Autodesk Inventor part; units mm, degrees
ref_plane "YZ Plane" through (0, 0, 0) normal (1, 0, 0) x (0, 1, 0)
ref_plane "XZ Plane" through (0, 0, 0) normal (0, 1, 0) x (-1, 0, 0)
ref_plane "XY Plane" through (0, 0, 0) normal (0, 0, 1) x (1, 0, 0)
sketch "Sketch1" plane through (0, 0, 0) normal (0, 0, 1) x (1, 0, 0)
  line L0 (0, 0) -> (31.75, 0)
  line L1 (31.75, 0) -> (31.75, 6.35)
  line L2 (31.75, 25.4) -> (28.575, 25.4) construction
  line L3 (0, 25.4) -> (0, 6.35) construction
  line L4 (0, 6.35) -> (3.175, 6.35)
  line L5 (3.175, 6.35) -> (3.175, 25.4)
  line L6 (28.575, 25.4) -> (28.575, 6.35)
  line L7 (28.575, 6.35) -> (31.75, 6.35)
  line L8 (0, 6.35) -> (0, 0)
  line L9 (3.175, 25.4) -> (0, 25.4) construction
  line L10 (28.575, 25.4) -> (3.175, 25.4)
  line L11 (31.75, 6.35) -> (31.75, 25.4) construction
  dimension "d0" = 31.75
  dimension "d1" = 25.4
  dimension "d2" = 6.35
  dimension "d3" = 3.175
extrude "Extrusion1" add sketch "Sketch1" along normal blind 98.425
sketch "Sketch2" plane through (3.175, 25.4, 0) normal (0, 1, 0) x (1, 0, 0)
  line L0 (0, -98.425) -> (25.4, -98.425)
  line L1 (25.4, 0) -> (25.4, -98.425)
  line L2 (25.4, 0) -> (0, 0)
  line L3 (0, 0) -> (0, -98.425)
  point P0 (-3.175, 0)
  point P1 (12.7, -85.725)
  point P2 (12.7, -12.7)
  dimension "d6" = 12.7
  dimension "d7" = 12.7
  dimension "d8" = 12.7
  dimension "d9" = 12.7
hole "Hole1" at (15.875, 25.4, 85.725) at (15.875, 25.4, 12.7) direction (0, -1, 0) diameter 6.35 end through all counterbore diameter 9.525 counterbore depth 6.35
properties part number "8 ball plastic slider"
Input: part model. Units: mm. Frame: model coordinates. A direction names the side the tool comes from. Coordinates: 2 decimals unless noted, no trailing zeros. Write each loop counter-clockwise with the first axis right and the second up, starting at its lowest first coordinate (ties: lowest second). Pieces come first, ordered by that corner, then holes. Notation, with made-up numbers: M -9,-2.75 L -3,-2.75 A14 ccw -3,5.25 Z; hole C -32.5,-12 d2. An arc over 180 degrees is marked long. Answer as a JSON object with one key per item and string values. Group by question number.
(1) Set-up query: faces 5 (the face through (18.77, 22.18, 8.92)), 6 (the face through (3.175, 16, 49)), 7 (the face through (16, 0, 49)), 8 (the face through (30, 6.35, 49)). Return all of +Z, -Z, +X, -X, +Y, -Y with unobstructed straight access to the full face (end or side cutting, diameter ignored); none if empty.
(2) Ray query, line 1 along Z through (x, y) = (15.5, 23) (3 decimals); line 2 along Z through (x, y) = (11.5, 24) (3 decimals); line 3 along X through (y, z) = (13.25, 12.7) (3 decimals). Return the intervals inside material, ascending. Write a range as [from, to].
(3) Section D-D on x = 30.5. Output: boundary loops of the cut face in (y, z) (3 decimals), plus the area to 3 significant figures.
(4) Section B-B on y = 5. Output: boundary loops of the cut face in (x, z) (3 decimals), plus the area to 3 significant figures.
(5) Section C-C on z = 25. Output: boundary loops of the cut face in (x, y) (3 decimals), plus the area to 3 significant figures.
(6) Contact query for flat-ended pins moving along their axis: P1, Ø1.5, axis at x = 8, y = 3, coming from the -Z side; P2, Ø5, axis at y = 22, z = 84, coming from the +X side (3 decimals); P3, Ø1.6, axis at x = 30, z = 70.5, coming from the +Y side; P4, Ø8.5, axis at x = 15.875, z = 12.7, coming from the +Y side. Output: stop coordinate, or through.
(7) Mould query, pull axis Z, two halves, no side actions, for faces 1 (the face through (31.75, 3, 49)), 2 (the face through (16, 13, 98.425)), 3 (the face through (18.773, 22.181, 81.946)), 4 (the face through (15.735, 9.392, 9.528)). Classes: pulls with the +Z half, pulls with the -Z half, needs draft (parallel to the pull), parting line crosses it, or undercut.
Result set:
{
 "1": {"face 5": "+Y", "face 6": "+Z, -Z, -X, +Y", "face 7": "+Z, -Z, +X, -X, -Y", "face 8": "+Z, -Z, +X, +Y"},
 "2": {"line 1": "z = [0, 7.952], [17.448, 80.977], [90.473, 98.425]", "line 2": "z = [0, 10.818], [14.582, 83.843], [87.607, 98.425]", "line 3": "x = [3.175, 12.7], [19.05, 28.575]"},
 "3": {"outline": "M 0,0 L 6.35,0 L 6.35,98.425 L 0,98.425 Z", "area": "625 mm2"},
 "4": {"outline": "M 0,0 L 31.75,0 L 31.75,98.425 L 0,98.425 Z; hole C 15.875,12.7 d6.35; hole C 15.875,85.725 d6.35", "area": "3,060 mm2"},
 "5": {"outline": "M 0,0 L 31.75,0 L 31.75,6.35 L 28.575,6.35 L 28.575,25.4 L 3.175,25.4 L 3.175,6.35 L 0,6.35 Z", "area": "685 mm2"},
 "6": {"P1": "stops at z = 0", "P2": "stops at x = 28.575", "P3": "stops at y = 6.35", "P4": "stops at y = 19.05"},
 "7": {"face 1": "needs draft", "face 2": "pulls with the +Z half", "face 3": "undercut", "face 4": "undercut"}
}
